from build123d import *

# Parameters (mm, degrees)
BOSS_EXTRUDE1_DEPTH = 68.724264069
BOSS_EXTRUDE2_DEPTH = 68.724264069
SKETCH2_R           = 1.8
CUT_EXTRUDE1_DEPTH  = 6
SKETCH3_R           = 1.8
CUT_EXTRUDE2_DEPTH  = 6
SKETCH5_W           = 68.724264069
SKETCH5_H           = 35.396446609
BOSS_EXTRUDE3_DEPTH = 3


with BuildPart() as part:
    # Sketch1 → Boss-Extrude1 (new body)
    with BuildSketch(Plane.XY.offset(10)):
        Polygon((24.362132034, 0), (24.362132034, 77.496446609), (63.362132034, 77.496446609), (63.362132034, 69.496446609), (32.362132034, 69.496446609), (32.362132034, 0), align=None)
    extrude(amount=-BOSS_EXTRUDE1_DEPTH)

    # Sketch4 → Boss-Extrude2 (add)
    with BuildSketch(Plane.XY.offset(10)):
        Polygon((32.362132034, 49.496446609), (32.362132034, 69.496446609), (52.362132034, 69.496446609), align=None)
    extrude(amount=-BOSS_EXTRUDE2_DEPTH)

    # Sketch2 → Cut-Extrude1 (cut)
    with BuildSketch(Plane(origin=(0, 77.496446609, 0), x_dir=(1, 0, 0), z_dir=(0, 1, 0))):
        with Locations(Location((58.362132034, 53.724264069, 0), (0, 0, 180))):
            Circle(SKETCH2_R)
        with Locations(Location((31.362132034, 53.724264069, 0), (0, 0, 180))):
            Circle(SKETCH2_R)
        with Locations(Location((58.362132034, -5, 0), (0, 0, 180))):
            Circle(SKETCH2_R)
        with Locations(Location((31.362132034, -5, 0), (0, 0, 180))):
            Circle(SKETCH2_R)
    extrude(amount=-CUT_EXTRUDE1_DEPTH, mode=Mode.SUBTRACT)

    # Sketch3 → Cut-Extrude2 (cut)
    with BuildSketch(Plane.ZY.offset(-24.362132034)):
        with Locations(Location((-53.724264069, 37, 0), (0, 0, 270))):
            Circle(SKETCH3_R)
        with Locations(Location((-53.724264069, 10, 0), (0, 0, 270))):
            Circle(SKETCH3_R)
        with Locations(Location((5, 10, 0), (0, 0, 270))):
            Circle(SKETCH3_R)
        with Locations(Location((5, 37, 0), (0, 0, 270))):
            Circle(SKETCH3_R)
    extrude(amount=-CUT_EXTRUDE2_DEPTH, mode=Mode.SUBTRACT)

    # Sketch5 → Boss-Extrude3 (add)
    with BuildSketch(Plane.ZY.offset(-24.362132034)):
        with Locations((-24.362132035, 59.748223305)):
            Rectangle(SKETCH5_W, SKETCH5_H)
    extrude(amount=BOSS_EXTRUDE3_DEPTH)


solid = part.part
Input: part model. Units: mm. Frame: model coordinates. A direction names the side the tool comes from. Give positions to 0.01 mm unless a question says otherwise; leave off trailing zeros. Loops run counter-clockwise (first coordinate to the right, second up) from the corner with the lowest first, then second, coordinate; pieces in that order, holes last. Notation, with made-up numbers: M -39,58.5 L -20,58.5 A32 ccw -20,94.5 Z; hole C 45,-7 d9. An arc over 180 degrees is marked long. Use one line per item in the form item = value.
1. Line query: L1, parallel to Z at x = 26.1, y = 10; L2, parallel to Y at x = 57, z = -2; L3, parallel to X at y = 30.5, z = -11.5. Output: solid intervals per line, ascending.
Numbers:
L1 = -58.72 to -55.52, -51.92 to 3.2, 6.8 to 10
L2 = 69.5 to 77.5
L3 = 24.36 to 32.36
2. First-contact query: pin 1 (5 mm diameter, centred on x = 52.5, z = -1, fed in from -Y); pin 2 (1.1 mm diameter, centred on x = 58, z = -54.5, fed in from +Y); pin 3 (1.1 mm diameter, centred on y = 10.5, z = 4, fed in from -X). Flat tips, straight axial feed; report the tip coordinate or a pass-through.
Numbers:
pin_1 = 67.13
pin_2 = 71.5
pin_3 = 30.36
3. Section query B-B, the plane z = 5. Return the cut outline in (x, y), and give its area (3 significant figures).
Numbers:
outline = M 21.36,42.05 L 24.36,42.05 L 24.36,38.8 L 30.36,38.8 L 30.36,35.2 L 24.36,35.2 L 24.36,11.8 L 30.36,11.8 L 30.36,8.2 L 24.36,8.2 L 24.36,0 L 32.36,0 L 32.36,49.5 L 52.36,69.5 L 63.36,69.5 L 63.36,77.5 L 60.16,77.5 L 60.16,71.5 L 56.56,71.5 L 56.56,77.5 L 33.16,77.5 L 33.16,71.5 L 29.56,71.5 L 29.56,77.5 L 24.36,77.5 L 24.36,77.45 L 21.36,77.45 Z
area = 1,090 mm²
4. Section query A-A, the plane y = 37. Return the cut outline in (x, z), and give its area (3 significant figures).
Numbers:
outline = M 24.36,-58.72 L 32.36,-58.72 L 32.36,10 L 24.36,10 L 24.36,6.8 L 30.36,6.8 L 30.36,3.2 L 24.36,3.2 L 24.36,-51.92 L 30.36,-51.92 L 30.36,-55.52 L 24.36,-55.52 Z
area = 507 mm²
5. Reachability of faces 4 (the face through (58, 69.496, -24)), 5 (the face through (56.7, 74.54, -54.41)), 6 (the face through (27.32, 10.39, -55.48)) from +Z, -Z, +X, -X, +Y, -Y: full face, straight path, thin tool, end or side. Return the list, or none.
Numbers:
face_4 = +Z, -Z, +X, -Y
face_5 = +Y
face_6 = -X
6. Section query C-C, the plane z = -39. Return the cut outline in (x, y).
Numbers:
outline = M 21.36,42.05 L 24.36,42.05 L 24.36,0 L 32.36,0 L 32.36,49.5 L 52.36,69.5 L 63.36,69.5 L 63.36,77.5 L 24.36,77.5 L 24.36,77.45 L 21.36,77.45 Z
7. Section query D-D, the plane x = 58.5. Return the cut outline in (y, z), and give its area (3 significant figures).
Numbers:
outline = M 69.5,-58.72 L 77.5,-58.72 L 77.5,-55.52 L 71.5,-55.52 L 71.5,-51.93 L 77.5,-51.93 L 77.5,3.21 L 71.5,3.21 L 71.5,6.79 L 77.5,6.79 L 77.5,10 L 69.5,10 Z
area = 507 mm²
8. Pull-direction query (Y, two-part tool) for faces 1 (the face through (30.362, 10, 5)), 2 (the face through (29.7, 74.54, -54.41)), 3 (the face through (44, 77.496, -24)); classes: released by +Y, released by -Y, zero draft, split by the parting line, or undercut.
Numbers:
face_1 = undercut
face_2 = zero draft
face_3 = released by +Y
